Read the model definition and answer for the solid it produces. Units are mm, in the model's axes. Coordinates: 2 decimals unless noted, no trailing zeros. Write each loop counter-clockwise with the first axis right and the second up, starting at its lowest first coordinate (ties: lowest second). Pieces come first, ordered by that corner, then holes.
1) Find the intervals of material crossed by line 1 (Y direction, x = 0, z = 4.05); line 2 (Y direction, x = 3.5, z = 4.65); line 3 (X direction, y = 3, z = 3.3), in increasing order.
2) The part is cut by section B-B (x = 0). Determine the outline of the cut face in (y, z).
3) Each of these flat-tipped pins is pushed along its axis until it touches: pin 1 Ø1.5 at (y, z) = (72.5, 1.5) entering from -X; pin 2 Ø1 at (x, z) = (-64.5, 3.5) entering from -Y; pin 3 Ø2 at (x, z) = (-53, 3.5) entering from +Y. Where does it stop, or does it pass through?
4) The part is cut by section C-C (z = 1.8). Determine the outline of the cut face in (x, y), then the cut area to 3 significant figures.
5) The part is cut by section D-D (y = 23). Determine the outline of the cut face in (x, z), then the cut area to 3 significant figures.
6) The part is cut by section A-A (y = 0). Determine the outline of the cut face in (x, z), then the cut area to 4 significant figures.
Autodesk Inventor part; units mm, degrees
ref_plane "YZ Plane" through (0, 0, 0) normal (1, 0, 0) x (0, 1, 0)
ref_plane "XZ Plane" through (0, 0, 0) normal (0, 1, 0) x (-1, 0, 0)
ref_plane "XY Plane" through (0, 0, 0) normal (0, 0, 1) x (1, 0, 0)
sketch "Sketch1" plane through (0, 0, 0) normal (0, 0, 1) x (1, 0, 0)
  circle A0 centre (0, 0) radius 100
  dimension "d8" = 200
extrude "Extrusion1" add sketch "Sketch1" along normal blind 5.5
sketch "Sketch2" plane through (0, 0, 5.5) normal (0, 0, 1) x (1, 0, 0)
  circle A0 centre (0, 23) radius 5
  point P0 (0, 0)
  dimension "d2" = 10
  dimension "d9" = 23
extrude "Extrusion2" cut sketch "Sketch2" against normal blind 100
sketch "Sketch3" plane through (0, 0, 0) normal (0, 0, -1) x (-1, 0, 0)
  circle A0 centre (0, 0) radius 5
  dimension "d5" = 10
extrude "Extrusion3" cut sketch "Sketch3" against normal blind 10
properties part number "pulley"
Reported:
1. line 1: y = -100 to -5, 5 to 18, 28 to 100
1. line 2: y = -99.94 to -3.57, 3.57 to 19.43, 26.57 to 99.94
1. line 3: x = -99.95 to -4, 4 to 99.95
2. outline: (-100, 0) - (-5, 0) - (-5, 5.5) - (-100, 5.5) - close; (5, 0) - (18, 0) - (18, 5.5) - (5, 5.5) - close; (28, 0) - (100, 0) - (100, 5.5) - (28, 5.5) - close
3. pin 1: stops at x = -69.66
3. pin 2: stops at y = -76.84
3. pin 3: stops at y = 85.42
4. outline: circle Ø200 at (0, 0); hole circle Ø10 at (0, 0); hole circle Ø10 at (0, 23)
4. area: 31,300 mm2
5. outline: (-97.32, 0) - (-5, 0) - (-5, 5.5) - (-97.32, 5.5) - close; (5, 0) - (97.32, 0) - (97.32, 5.5) - (5, 5.5) - close
5. area: 1,020 mm2
6. outline: (-100, 0) - (-5, 0) - (-5, 5.5) - (-100, 5.5) - close; (5, 0) - (100, 0) - (100, 5.5) - (5, 5.5) - close
6. area: 1,045 mm2
